Input: part model. Units: mm. Frame: model coordinates. A direction names the side the tool comes from. Round coordinates to 2 decimals unless told otherwise and drop trailing zeros. Loops run counter-clockwise (first coordinate to the right, second up) from the corner with the lowest first, then second, coordinate; pieces in that order, holes last. Notation, with made-up numbers: M 60.5,64 L 92.5,64 A22 cw 92.5,70 Z; hole C 64.25,25.25 d2. An arc over 180 degrees is marked long. Put each result on its own line as item: value. Start each with the question number.
1) Line query: probe 1 along X at (y, z) = (0, 2.3); probe 2 along Z at (x, y) = (19.5, 4.25); probe 3 along Y at (x, z) = (-13.5, -9.5). Output: solid intervals per line, ascending.
2) Section A-A on z = -10.25. Output: boundary loops of the cut face in (x, y), plus the area to 3 significant figures.
3) Section B-B on x = -0.5. Output: boundary loops of the cut face in (y, z), plus the area to 3 significant figures.
4) Pin query (flat end, axial travel): pin 1 (8 mm diameter, centred on x = -2.5, z = -10.5, fed in from -Y); pin 2 (6 mm diameter, centred on x = -3.5, y = 2, fed in from -Z); pin 3 (6 mm diameter, centred on x = 11, y = -2.5, fed in from -Z); pin 4 (3 mm diameter, centred on x = -16, y = 0, fed in from +Z). Return the tip coordinate at first contact, or that it passes through.
5) Section C-C on y = 0. Output: boundary loops of the cut face in (x, z).
6) Section D-D on z = 3.5. Output: boundary loops of the cut face in (x, y).
7) Draft query along X for faces 4 (the face through (-9.01, 1.5, 2.04)), 5 (the face through (-6, -10, 0)), 6 (the face through (-7.5, 0, -8)). Return one class per face: +X half, -X half, draft (parallel to the pull), parting line (faces both ways), or undercut.
8) Reachability of faces 1 (the face through (-12, -2, -1)), 2 (the face through (-19.548, 7.004, 3.732)), 3 (the face through (9, 0, 0)) from +Z, -Z, +X, -X, +Y, -Y: full face, straight path, thin tool, end or side. Return the list, or none.
from build123d import *

# Parameters (mm, degrees)
SKETCH1_W       = 45
SKETCH1_H       = 20
EXTRUDE1_DEPTH  = 5
SKETCH2_W       = 15
SKETCH2_H       = 20
EXTRUDE2_DEPTH  = 13
SKETCH3_R       = 5
EXTRUDE3_DEPTH  = 6
SKETCH4_R       = 2.5
EXTRUDE4_DEPTH  = 16
FILLET1_R       = 5
CHAMFER1_SIZE   = 4.330127019
CHAMFER1_SIZE_2 = 2.5
FILLET2_R       = 3


with BuildPart() as part:
    # Sketch1 → Extrude1 (new body)
    with BuildSketch(Plane.XY):
        Rectangle(SKETCH1_W, SKETCH1_H)
    extrude(amount=EXTRUDE1_DEPTH)

    # Sketch2 → Extrude2 (add)
    with BuildSketch(Plane(origin=(0, 0, 0), x_dir=(-1, 0, 0), z_dir=(0, 0, -1))):
        with Locations((15, 0)):
            Rectangle(SKETCH2_W, SKETCH2_H)
    extrude(amount=EXTRUDE2_DEPTH)

    # Sketch3 → Extrude3 (cut)
    with BuildSketch(Plane.XY.offset(5)):
        with Locations((-13.77840955, 0)):
            Circle(SKETCH3_R)
    extrude(amount=-EXTRUDE3_DEPTH, mode=Mode.SUBTRACT)

    # Sketch4 → Extrude4 (cut)
    with BuildSketch(Plane.XY.offset(-1)):
        with Locations((-13.77840955, 0)):
            Circle(SKETCH4_R)
    extrude(amount=-EXTRUDE4_DEPTH, mode=Mode.SUBTRACT)

    # Fillet1
    fillet1_edges = [part.edges().sort_by_distance(p)[0] for p in [
        (-22.5, 10, -4),
        (-22.5, -10, -4),
    ]]
    fillet(fillet1_edges, radius=FILLET1_R)

    # Chamfer1
    # the kernel refuses this chamfer: 4.330127019, 2.5 mm, written as the material it takes off along each edge
    with BuildSketch(Plane(origin=(-17.5, 10, 5), x_dir=(0, -0.999813220622208, 0.01932676561270069), z_dir=(1, 0, 0))) as chamfer1_piece_1:
        Polygon((CHAMFER1_SIZE * 0.999813220604, CHAMFER1_SIZE * 0.0193267656124), (-CHAMFER1_SIZE_2 * 0.0193267656127, CHAMFER1_SIZE_2 * 0.999813220622), (0, 0), align=None)
    extrude(amount=51.202409926, mode=Mode.SUBTRACT)
    with BuildSketch(Plane(origin=(33.702409926, -10, 5), x_dir=(0, -0.05789386240267114, -0.9983227437537926), z_dir=(-1, 0, 0))) as chamfer1_piece_2:
        Polygon((CHAMFER1_SIZE_2 * 0.998322743754, -CHAMFER1_SIZE_2 * 0.0578938624027), (-CHAMFER1_SIZE * 0.0578938624016, -CHAMFER1_SIZE * 0.998322743736), (0, 0), align=None)
    extrude(amount=51.202409926, mode=Mode.SUBTRACT)
    with BuildSketch(Plane(origin=(-22.5, -5, 5), x_dir=(0.999813220622208, 0, 0.01932676561270069), z_dir=(0, 1, 0))) as chamfer1_piece_3:
        Polygon((CHAMFER1_SIZE * 0.999813220604, CHAMFER1_SIZE * 0.0193267656124), (-CHAMFER1_SIZE_2 * 0.0193267656127, CHAMFER1_SIZE_2 * 0.999813220622), (0, 0), align=None)
    extrude(amount=10, mode=Mode.SUBTRACT)
    with BuildSketch(Plane(origin=(-17.5, 5, 5), x_dir=(-1, 0, 0), z_dir=(0, -1, 0))) as chamfer1_piece_4:
        Polygon((5 - CHAMFER1_SIZE, 0), (5, CHAMFER1_SIZE_2), (5, 0), align=None)
    revolve(axis=Axis((-17.5, 5, 5), (0, 0, -1)), revolution_arc=90, mode=Mode.SUBTRACT)
    with BuildSketch(Plane(origin=(-17.5, -5, 5), x_dir=(0, -1, 0), z_dir=(1, 0, 0))) as chamfer1_piece_5:
        Polygon((5 - CHAMFER1_SIZE, 0), (5, CHAMFER1_SIZE_2), (5, 0), align=None)
    revolve(axis=Axis((-17.5, -5, 5), (0, 0, -1)), revolution_arc=90, mode=Mode.SUBTRACT)

    # Fillet2
    fillet2_edges = [part.edges().sort_by_distance(p)[0] for p in [
        (-7.5, 0, 0),
    ]]
    fillet(fillet2_edges, radius=FILLET2_R)


solid = part.part
Geometry results:
1. probe 1: x = -22.5 to -18.78, -8.78 to 22.5
1. probe 2: z = 0 to 5
1. probe 3: y = -10 to -2.48, 2.48 to 10
2. outline: M -22.5,-5 A5 ccw -17.5,-10 L -7.5,-10 L -7.5,10 L -17.5,10 A5 ccw -22.5,5 Z; hole C -13.78,0 d5
2. area: 270 mm²
3. outline: M -10,0 L 10,0 L 10,2.5 L 5.67,5 L -5.67,5 L -10,2.5 Z
3. area: 89.2 mm²
4. pin 1: passes through
4. pin 2: stops at z = -0.76
4. pin 3: stops at z = 0
4. pin 4: stops at z = -1
5. outline: M -22.5,-13 L -16.28,-13 L -16.28,-1 L -18.78,-1 L -18.78,4.65 L -22.5,2.5 Z; M -11.28,-13 L -7.5,-13 L -7.5,-3 A3 cw -4.5,0 L 22.5,0 L 22.5,5 L -8.78,5 L -8.78,-1 L -11.28,-1 Z
6. outline: M -20.77,-5 A3.27 ccw -17.5,-8.27 L 22.5,-8.27 L 22.5,8.27 L -17.5,8.27 A3.27 ccw -20.77,5 Z; hole C -13.78,0 d10
7. face 4: undercut
7. face 5: draft
7. face 6: +X half
8. face 1: +Z
8. face 2: +Z, -X, +Y
8. face 3: -Z, +X, +Y, -Y
